from build123d import *

# Parameters (mm, degrees)
F0_W      = 108
F0_H      = 130
F1_DEPTH  = 110
F2_R      = 6.5
F3_DEPTH  = 110.001
F4_W      = 108
F4_H      = 95
F5_DEPTH  = 70
F6_W      = 110
F6_H      = 25
F7_DEPTH  = 25
F8_R      = 6.5
F9_DEPTH  = 5
F10_R     = 4.99999
F11_R     = 10
F12_DEPTH = 20
F13_R     = 10
F14_DEPTH = 20
F15_W     = 20
F15_H     = 55
F15_W_2   = 44
F15_H_2   = 20
F16_DEPTH = 5


# Not quite as in the source:
# - a fillet or chamfer is up to 0.001 mm smaller than in the source, because OpenCascade refuses the exact size


with BuildPart() as f1:
    # F0 (on Right) → F1 (new body)
    with BuildSketch(Plane.YZ):
        Rectangle(F0_W, F0_H)
    extrude(amount=-F1_DEPTH)

    # F2 (on face) → F3 (cut, through all)
    with BuildSketch(Plane(origin=(-110, 0, 0), x_dir=(0, -1, 0), z_dir=(-1, 0, 0))):
        with Locations((-42, 47)):
            Circle(F2_R)
        with Locations((42, 47)):
            Circle(F2_R)
        with Locations((-42, -47)):
            Circle(F2_R)
        with Locations((42, -47)):
            Circle(F2_R)
    extrude(amount=-F3_DEPTH, mode=Mode.SUBTRACT)

    # F4 (on face) → F5 (cut)
    with BuildSketch(Plane(origin=(-110, 0, 0), x_dir=(0, -1, 0), z_dir=(-1, 0, 0))):
        with Locations((0, 17.5)):
            Rectangle(F4_W, F4_H)
    extrude(amount=-F5_DEPTH, mode=Mode.SUBTRACT)

    # F6 (on face) → F7 (cut)
    with BuildSketch(Plane(origin=(0, 0, -65), x_dir=(1, 0, 0), z_dir=(0, 0, -1))):
        with Locations((-55, -11.5)):
            Rectangle(F6_W, F6_H)
    extrude(amount=-F7_DEPTH, mode=Mode.SUBTRACT)

    # F8 (on face) → F9 (cut)
    with BuildSketch(Plane(origin=(-110, 0, 0), x_dir=(0, -1, 0), z_dir=(-1, 0, 0))):
        Polygon((-24, -30), (-24, -40), (1, -40), (1, -65), (54, -65), (54, -30), align=None)
        with Locations((42, -47)):
            Circle(F8_R, mode=Mode.SUBTRACT)
    extrude(amount=-F9_DEPTH, mode=Mode.SUBTRACT)

    # F10 (radius 5 in the source; OpenCascade refuses exactly that, so slightly less here)
    f10_edges = [f1.edges().sort_by_distance(p)[0] for p in [
        (-105, 24, -35),
    ]]
    fillet(f10_edges, radius=F10_R)

    # F11 (on face) → F12 (cut)
    with BuildSketch(Plane(origin=(-40, 0, 0), x_dir=(0, -1, 0), z_dir=(-1, 0, 0))):
        with Locations((-42, 47)):
            Circle(F11_R)
        with Locations((42, 47)):
            Circle(F11_R)
    extrude(amount=-F12_DEPTH, mode=Mode.SUBTRACT)

    # F13 (on face) → F14 (cut)
    with BuildSketch(Plane(origin=(-110, 0, 0), x_dir=(0, -1, 0), z_dir=(-1, 0, 0))):
        with Locations((-42, -47)):
            Circle(F13_R)
        with Locations((42, -47)):
            Circle(F13_R)
    extrude(amount=-F14_DEPTH, mode=Mode.SUBTRACT)

    # F15 (on face) → F16 (cut)
    with BuildSketch(Plane.YZ):
        with Locations((0, 37.5)):
            Rectangle(F15_W, F15_H)
        with Locations((32, 0)):
            Rectangle(F15_W_2, F15_H_2)
        Rectangle(F15_W, F15_H_2)
        with Locations((-32, 0)):
            Rectangle(F15_W_2, F15_H_2)
        with Locations((0, -37.5)):
            Rectangle(F15_W, F15_H)
    extrude(amount=-F16_DEPTH, mode=Mode.SUBTRACT)


solid = f1.part
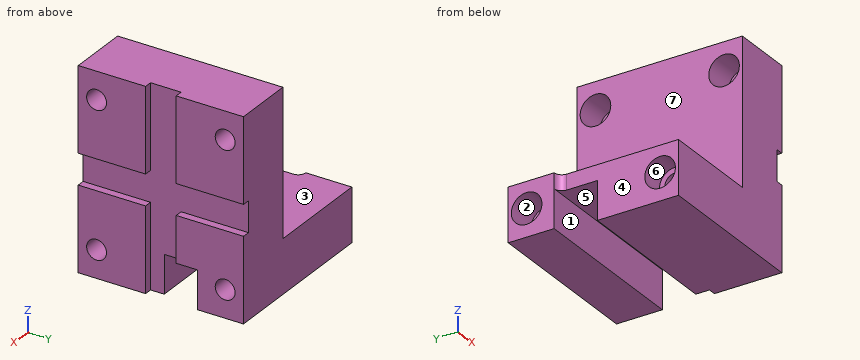
Work out the finished part from the listing and answer in its coordinate system (mm). Face numbers are marked on the shaded views. A direction names the side the tool comes from. Round coordinates to 2 decimals unless told otherwise and drop trailing zeros. Order: outer loops, then holes, each group sorted by start corner. A loop starts at its lowest first (then second) coordinate and runs counter-clockwise, first axis right, second up. Notation, with made-up numbers: M -5.5,-27 L 46.5,-27 A26 cw 46.5,6 Z; hole C 20,37 d7. An arc over 180 degrees is marked long. One line per item, written item: value.
Q1. Flat-ended cylindrical pins translate along their axes: pin 1 (10 mm diameter, centred on y = 45, z = 46, fed in from -X); pin 2 (3 mm diameter, centred on y = 21, z = 2.5, fed in from +X); pin 3 (1.5 mm diameter, centred on y = 4, z = 5, fed in from -X). Find the tip coordinate at first contact, or state that the pin passes through.
Derived:
pin 1: x = -20
pin 2: x = -5
pin 3: x = -40
Q2. Find section B-B on z = 47. Write down the section's boundary in (x, y).
Derived:
outline: M -40,-54 L 0,-54 L 0,-48.5 L -20,-48.5 L -20,-52 L -40,-52 Z; M -40,-32 L -20,-32 L -20,-35.5 L 0,-35.5 L 0,-10 L -5,-10 L -5,10 L 0,10 L 0,35.5 L -20,35.5 L -20,32 L -40,32 Z; M -40,52 L -20,52 L -20,48.5 L 0,48.5 L 0,54 L -40,54 Z
Q3. Find section D-D on z = -47. Write down the section's boundary in (x, y).
Derived:
outline: M -110,24 L 0,24 L 0,35.5 L -90,35.5 L -90,32 L -110,32 Z; M -110,52 L -90,52 L -90,48.5 L 0,48.5 L 0,54 L -110,54 Z; M -105,-54 L 0,-54 L 0,-48.5 L -90,-48.5 L -90,-52 L -105,-52 Z; M -105,-32 L -90,-32 L -90,-35.5 L 0,-35.5 L 0,-10 L -5,-10 L -5,-1 L -105,-1 Z
Q4. Find section A-A on y = 42. Write down the section's boundary in (x, z).
Derived:
outline: M -110,-65 L 0,-65 L 0,-53.5 L -90,-53.5 L -90,-57 L -110,-57 Z; M -110,-37 L -90,-37 L -90,-40.5 L 0,-40.5 L 0,-10 L -5,-10 L -5,10 L 0,10 L 0,40.5 L -20,40.5 L -20,37 L -40,37 L -40,-30 L -110,-30 Z; M -40,57 L -20,57 L -20,53.5 L 0,53.5 L 0,65 L -40,65 Z
Q5. For the marked faces 1, 2, 3 and 4, determine the directions among +Z, -Z, +X, -X, +Y, -Y from which every point of the face is accessible in a straight line to the end or side of a thin tool.
Derived:
face 1: -Z, +X, -X
face 2: -X
face 3: +Z, -X, +Y, -Y
face 4: +Z, -Z, -X, -Y
Q6. Determine the mould class of the marked faces 5, 6 and 7 for opening direction Z: released by +Z, released by -Z, zero draft, split by the parting line, or undercut.
Derived:
face 5: released by -Z
face 6: undercut
face 7: zero draft
Q7. Find section C-C on x = -67.5. Write down the section's boundary in (y, z), then the cut area to 3 significant figures.
Derived:
outline: M -54,-65 L -1,-65 L -1,-40 L 24,-40 L 24,-65 L 54,-65 L 54,-30 L -54,-30 Z; hole C -42,-47 d13; hole C 42,-47 d13
area: 2,890 mm²
Q8. Straight lines are drawn through the part: line 1 (Z direction, x = -9, y = 42); line 2 (Z direction, x = -32, y = 42); line 3 (Y direction, x = -51.5, z = -44.5). For each, find the intervals that lie inside material, in ascending order.
Derived:
line 1: -65 to -53.5, -40.5 to 40.5, 53.5 to 65
line 2: -65 to -53.5, -40.5 to 37, 57 to 65
line 3: -54 to -48, -36 to -1, 24 to 36, 48 to 54
